```python
from build123d import *

# Parameters (mm, degrees)
BOSS_EXTRUDE1_DEPTH = 354.0125
SKETCH2_R           = 2.2225
SKETCH2_R_2         = 3.175
CUT_EXTRUDE1_DEPTH  = 1.27


with BuildPart() as part:
    # Sketch1 → Boss-Extrude1 (new body)
    with BuildSketch(Plane.XY):
        Polygon((0, 0), (0, -11.5316), (45.2628, -11.5316), (45.2628, 0), (43.9928, 0), (43.9928, -10.2616), (1.27, -10.2616), (1.27, 0), align=None)
    extrude(amount=BOSS_EXTRUDE1_DEPTH)

    # Sketch2 → Cut-Extrude1 (cut)
    with BuildSketch(Plane(origin=(0, -11.5316, 0), x_dir=(-1, 0, 0), z_dir=(0, -1, 0))):
        with Locations((-22.6314, -19.1897)):
            Circle(SKETCH2_R)
        with Locations((-22.6314, -80.391)):
            Circle(SKETCH2_R)
        with Locations((-22.6314, -319.2145)):
            Circle(SKETCH2_R_2)
    extrude(amount=-CUT_EXTRUDE1_DEPTH, mode=Mode.SUBTRACT)


solid = part.part
```
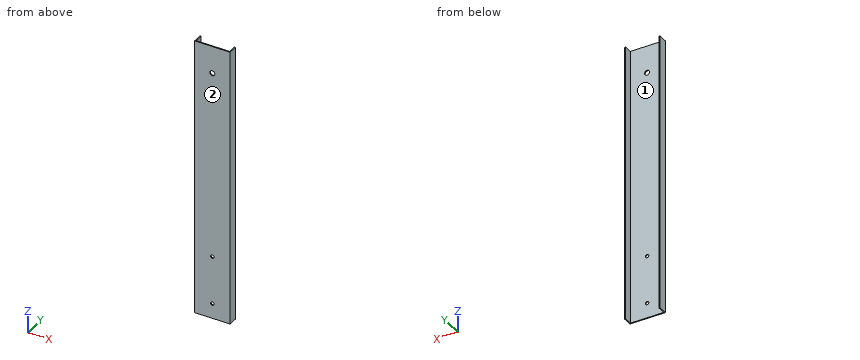
Model file for the job. Use its own axes, mm. Face numbers are marked on the shaded views. A direction names the side the tool comes from. Give positions to 0.01 mm unless a question says otherwise; leave off trailing zeros. Order: outer loops, then holes, each group sorted by start corner. A loop starts at its lowest first (then second) coordinate and runs counter-clockwise, first axis right, second up.
1) Saw through at B-B, the plane z = 49.5. Write the cut outline in (x, y).
2) 3-axis set-ups, long thin cutter, end or side, ignore diameter. For the marked faces 1 and 2: which of +Z, -Z, +X, -X, +Y, -Y reach the whole face in a straight line?
3) Saw through at C-C, the plane x = 9. Write the cut outline in (y, z).
4) Pin check, flat tips, straight feed: pin 1 (1 mm diameter, centred on y = -8.5, z = 89.5, fed in from -X); pin 2 (2.5 mm diameter, centred on x = 22.63, z = 80.39, fed in from +Y); pin 3 (8.5 mm diameter, centred on x = 22.63, z = 319.21, fed in from +Y). Stop position of each tip, or through.
5) Saw through at A-A, the plane y = -4.25. Write the cut outline in (x, z), then the cut area to 3 significant figures.
6) Wall check: probe 1 along X at (y, z) = (-7.5, 221); probe 2 along Y at (x, z) = (43, 71.5). Give the ranges that are in metal, low to high.
Computed:
1. outline: (0, -11.53) - (45.26, -11.53) - (45.26, 0) - (43.99, 0) - (43.99, -10.26) - (1.27, -10.26) - (1.27, 0) - (0, 0) - close
2. face 1: +Z, -Z, +Y
2. face 2: +Z, -Z, +X, -X, -Y
3. outline: (-11.53, 0) - (-10.26, 0) - (-10.26, 354.01) - (-11.53, 354.01) - close
4. pin 1: stops at x = 0
4. pin 2: passes through
4. pin 3: stops at y = -10.26
5. outline: (0, 0) - (1.27, 0) - (1.27, 354.01) - (0, 354.01) - close; (43.99, 0) - (45.26, 0) - (45.26, 354.01) - (43.99, 354.01) - close
5. area: 899 mm2
6. probe 1: x = 0 to 1.27, 43.99 to 45.26
6. probe 2: y = -11.53 to -10.26
